Can you work these out from the model? Positions are in its coordinate system, mm. A direction names the side the tool comes from. Coordinates: 2 decimals unless noted, no trailing zeros. Loops run counter-clockwise (first coordinate to the right, second up) from the corner with the lowest first, then second, coordinate; pieces in that order, holes last.
```python
from build123d import *

# Parameters (mm, degrees)
F0_W     = 34
F0_H     = 4
F1_DEPTH = 7
F2_R     = 1.99999


# Not quite as in the source:
# - a fillet or chamfer is up to 0.001 mm smaller than in the source, because OpenCascade refuses the exact size


with BuildPart() as f1:
    # F0 (on Top) → F1 (new body)
    with BuildSketch(Plane.XY):
        Polygon((48, 0), (0, 0), (0, -4), (7, -4), (41, -4), (48, -4), align=None)
        with Locations((24, -6)):
            Rectangle(F0_W, F0_H)
    extrude(amount=F1_DEPTH)

    # F2 (radius 2 in the source; OpenCascade refuses exactly that, so slightly less here)
    f2_edges = [f1.edges().sort_by_distance(p)[0] for p in [
        (48, -4, 3.5),
        (48, 0, 3.5),
        (0, -4, 3.5),
        (0, 0, 3.5),
    ]]
    fillet(f2_edges, radius=F2_R)


solid = f1.part
```
Item 1: I'm going to push flat-ended pins straight in: P1, Ø4, axis at x = 3.5, z = 4.5, coming from the -Y side; P2, Ø1.2, axis at y = -6, z = 2.5, coming from the +X side. Where does each tip first touch, or does it pass through?
Results are:
P1: stops at y = -4
P2: stops at x = 41
Item 2: On a 3-axis mill with a long thin cutter (end or side, diameter ignored), from which of +Z, -Z, +X, -X, +Y, -Y can I reach the whole of each face in a straight line? I mean faces 1 (the face through (43, -4, 3)), 2 (the face through (7, -6, 3)), 3 (the face through (0.6, -0.57, 3.55)). Say none if no direction works.
Results are:
face 1: +Z, -Z, +X, -Y
face 2: +Z, -Z, -X, -Y
face 3: +Z, -Z, -X, +Y
Item 3: Suppose I cut it at C-C, the plane y = -3.25. Please give me the cut outline in (x, z), plus the area to 3 significant figures.
Results are:
outline: (0.44, 0) - (47.56, 0) - (47.56, 7) - (0.44, 7) - close
area: 330 mm2
Item 4: Suppose I cut it at B-B, the plane y = -5.5. Please give me the cut outline in (x, z).
Results are:
outline: (7, 0) - (41, 0) - (41, 7) - (7, 7) - close
Item 5: I need wall thicknesses on line 1 along Y through (x, z) = (2, 2.75); line 2 along X through (y, z) = (-6, 1); line 3 along X through (y, z) = (-1.5, 6.25). Which ranges of each line are inside material? Lowest first, please.
Results are:
line 1: y = -4 to 0
line 2: x = 7 to 41
line 3: x = 0.06 to 47.94
